```python
from build123d import *

# Parameters (mm, degrees)
BOSS_EXTRUDE1_DEPTH = 4
BOSS_EXTRUDE1_DRAFT = 1
SHELL1_T            = -0.5
SKETCH2_R           = 2
BOSS_EXTRUDE2_DEPTH = 5.5
BOSS_EXTRUDE2_TAPER = 1.5
CIRPATTERN1_COUNT   = 4
SKETCH4_R           = 1.605977431
CUT_EXTRUDE1_DEPTH  = 5.5
CUT_EXTRUDE1_DRAFT  = 1.5


with BuildPart() as part:
    # Sketch1 → Boss-Extrude1 (with draft: the straight prism first)
    with BuildSketch(Plane(origin=(0, 0, 0), x_dir=(1, 0, 0), z_dir=(0, 1, 0))):
        with BuildLine():
            Line((-7.5, -6.375), (7.5, -6.375))
            ThreePointArc((7.5, -6.375), (8.207106781, -6.082106781), (8.5, -5.375))
            Line((8.5, -5.375), (8.5, 5.375))
            ThreePointArc((8.5, 5.375), (8.207106781, 6.082106781), (7.5, 6.375))
            Line((7.5, 6.375), (-7.5, 6.375))
            ThreePointArc((-7.5, 6.375), (-8.207106781, 6.082106781), (-8.5, 5.375))
            Line((-8.5, 5.375), (-8.5, -5.375))
            ThreePointArc((-8.5, -5.375), (-8.207106781, -6.082106781), (-7.5, -6.375))
        make_face()
    extrude(amount=-BOSS_EXTRUDE1_DEPTH)
    # Boss-Extrude1: the draft: its side faces are tilted about the plane it starts from
    boss_extrude1_sides = [part.faces().sort_by_distance(p)[0] for p in [
        (0, -2, 6.375),
        (8.207106781, -2, 6.082106781),
        (8.5, -2, 0),
        (8.207106781, -2, -6.082106781),
        (0, -2, -6.375),
        (-8.207106781, -2, -6.082106781),
        (-8.5, -2, 0),
        (-8.207106781, -2, 6.082106781),
    ]]
    draft(boss_extrude1_sides, Plane(origin=(0, 0, 0), x_dir=(1, 0, 0), z_dir=(0, 1, 0)), BOSS_EXTRUDE1_DRAFT)

    # Shell1
    shell1_openings = [part.faces().sort_by_distance(p)[0] for p in [
        (0, -4, 0),
    ]]
    offset(amount=SHELL1_T, openings=shell1_openings, kind=Kind.INTERSECTION)

    # Sketch2 → Boss-Extrude2 (add)
    with BuildSketch(Plane.XZ.offset(0.5)):
        Circle(SKETCH2_R)
    extrude(amount=BOSS_EXTRUDE2_DEPTH, taper=BOSS_EXTRUDE2_TAPER)

    # Rib1: read off the stored shape, not the designer's step
    # Rib1: loft between two sections, ruled curve by curve
    rib1_from = [
        Edge.make_line((1.98200868, -0.5, 0.267659472), (3, -0.5, 0.25)),
        Edge.make_line((1.98200868, -0.5, -0.267659472), (3, -0.5, -0.25)),
        Edge.make_line((3, -0.5, -0.25), (3, -0.5, 0.25)),
        Edge.make_line((1.98200868, -0.5, -0.267659472), (1.98200868, -0.5, 0.267659472)),
    ]
    rib1_to = [
        Edge.make_line((1.837744445, -6, 0.259514127), (2.386192277, -6, 0.25)),
        Edge.make_line((1.837744445, -6, -0.259514127), (2.386192277, -6, -0.25)),
        Edge.make_line((2.386192277, -6, -0.25), (2.386192277, -6, 0.25)),
        Edge.make_line((1.837744445, -6, -0.259514127), (1.837744445, -6, 0.259514127)),
    ]
    rib1 = Solid(Shell([*[Face.make_surface_from_curves(rib1_from[k], rib1_to[k]) for k in range(4)], Face(Wire(rib1_from)), Face(Wire(rib1_to))]))
    add(rib1)

    # CirPattern1: Rib1 ×4 about axis
    cirpattern1_axis = Axis((0, 0, 0), (0, 1, 0))
    for i in range(1, CIRPATTERN1_COUNT):
        add(rib1.rotate(cirpattern1_axis, i * 360 / CIRPATTERN1_COUNT))


with BuildPart() as cut_extrude1_tool:
    # Sketch4 → Cut-Extrude1 (with draft: the straight prism first)
    with BuildSketch(Plane.XZ.offset(6)):
        Circle(SKETCH4_R)
    extrude(amount=-CUT_EXTRUDE1_DEPTH)
    # Cut-Extrude1: the draft: its side faces are tilted about the plane it starts from
    cut_extrude1_sides = [cut_extrude1_tool.faces().sort_by_distance(p)[0] for p in [
        (-1.605977431, -3.25, 0),
    ]]
    draft(cut_extrude1_sides, Plane.XZ.offset(6), CUT_EXTRUDE1_DRAFT)


with BuildPart() as part_1:
    add(part.part)

    # Cut-Extrude1: cut by cut_extrude1_tool
    add(cut_extrude1_tool.part, mode=Mode.SUBTRACT)


solid = part_1.part
```
The listing builds one solid part. Answer for the finished solid, in the listing's coordinates (mm). A direction names the side the tool comes from. Coordinates: 2 decimals unless noted, no trailing zeros. Write each loop counter-clockwise with the first axis right and the second up, starting at its lowest first coordinate (ties: lowest second). Pieces come first, ordered by that corner, then holes.
Q1. The mould has two halves that part along X. Classify faces 5 (the flat face through (0, -0.5, 0)), 6 (the conical face through (-8.24, -1.97, 6.1)), 7 (the conical face through (8.223, -1.972, 6.114)): released by +X, released by -X, zero draft, split by the parting line, or undercut.
Returned:
face 5: undercut
face 6: released by -X
face 7: released by +X
Q2. Section A-A, the plane x = -3.25 is taken. Write down the section's boundary in (y, z) (3 decimals), then the cut area to 3 significant figures.
Returned:
outline: (-4, -6.445) - (0, -6.375) - (0, 6.375) - (-4, 6.445) - (-4, 5.945) - (-0.5, 5.884) - (-0.5, -5.884) - (-4, -5.945) - close
area: 9.88 mm2
Q3. Given P1, Ø1, axis at x = 0, z = 0, coming from the -Y side; P2, Ø1.5, axis at y = -2, z = 2, coming from the +X side, each flat-ended and moving along its own axis, determine where each tip first touches the part or whether it passes through.
Returned:
P1: stops at y = -0.5
P2: stops at x = 8.55
Q4. Which of the six approach directions +Z, -Z, +X, -X, +Y, -Y give full straight-line access (tool end or side, diameter ignored) to faces 1 (the conical face through (-8.223, -1.972, -6.114)), 2 (the conical face through (-1.375, -3.288, -1.35)), 3 (the flat face through (2, -6, 0)), 4 (the conical face through (8.24, -1.97, -6.1))?
Returned:
face 1: -Z, -X, +Y
face 2: -Y
face 3: +Z, -Z, +X, -X, -Y
face 4: -Z, +X, +Y
Q5. Section B-B, the plane y = -2.25 is taken. Give the number of separate pieces and of enclosed holes in the cut face, then the cut area to 3 significant figures.
Returned:
separate pieces: 2
enclosed holes: 2
area: 32.9 mm2
Q6. Find the intervals of material crossed by line 1 along Z through (x, y) = (-2.25, -2.25); line 2 along X through (y, z) = (-1.25, 2.75); line 3 along Y through (x, z) = (6.25, -0.5), in increasing order.
Returned:
line 1: z = -6.41 to -5.91, -0.26 to 0.26, 5.91 to 6.41
line 2: x = -8.52 to -8.02, -0.25 to 0.25, 8.02 to 8.52
line 3: y = -0.5 to 0
